Geometry: final body of the model. Coordinates: model frame, mm. Give positions to 0.01 mm unless a question says otherwise; leave off trailing zeros. Write each loop counter-clockwise with the first axis right and the second up, starting at its lowest first coordinate (ties: lowest second). Pieces come first, ordered by that corner, then holes.
Autodesk Fusion 360 part; units mm, degrees
sketch "Sketch1" plane through (0, 0, 0) normal (0, 0, 1) x (1, 0, 0)
  line L0 (0, 1.5) -> (-2, 1.5)
  line L1 (0, 1.5) -> (2, 1.5)
  arc A0 (-2, 1.5) -> (-2, -1.5) centre (0, 0) ccw
  arc A1 (2, -1.5) -> (2, 1.5) centre (0, 0) ccw
  circle A2 centre (0, 0) radius 3.5
  line L2 (-2, -1.5) -> (2, -1.5)
  dimension "d2" = 5
  dimension "d3" = 1.5
  dimension "d5" = 7
extrude "Extrude1" add sketch "Sketch1" along normal blind 20 contours L0 L1 A0 A1 L2
sketch "Sketch2" plane through (0, 0, 0) normal (0, 0, 1) x (1, 0, 0)
Q1. Section B-B on y = 0.7. Output: boundary loops of the cut face in (x, z).
Filled sheet:
outline: (-2.4, 0) - (2.4, 0) - (2.4, 20) - (-2.4, 20) - close
Q2. Section A-A on z = 7.25. Output: boundary loops of the cut face in (x, y).
Filled sheet:
outline: (-2, -1.5) - (2, -1.5) arc R2.5 ccw to (2, 1.5) - (-2, 1.5) arc R2.5 ccw to start
Q3. Ray query, line 1 along X through (y, z) = (0.1, 18.25); line 2 along Y through (x, z) = (-2.3, 3.5); line 3 along X through (y, z) = (0.75, 4.25). Return the intervals inside material, ascending.
Filled sheet:
line 1: x = -2.5 to 2.5
line 2: y = -0.98 to 0.98
line 3: x = -2.38 to 2.38
